Read the model definition and answer for the solid it produces. Units are mm, in the model's axes. Give positions to 0.01 mm unless a question says otherwise; leave off trailing zeros. Loops run counter-clockwise (first coordinate to the right, second up) from the corner with the lowest first, then second, coordinate; pieces in that order, holes last. Notation, with made-up numbers: (37, -6.75) -> (47, -6.75) arc R23 ccw to (47, 7.25) -> close; hole circle Ø4 at (5, 47). An arc over 180 degrees is marked (long way). One line per item, written item: value. Start each with the question number.
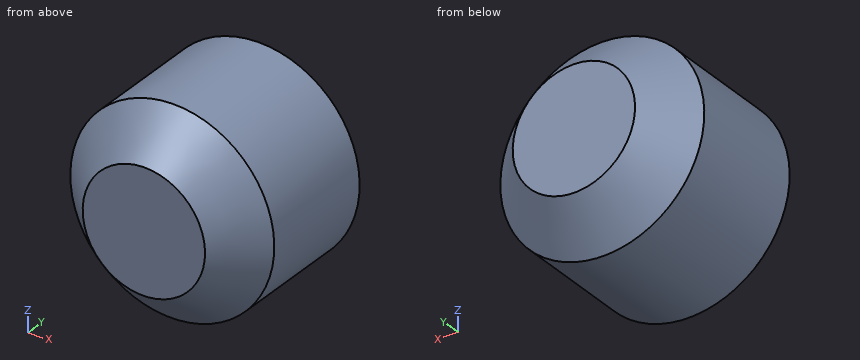
from build123d import *

# Parameters (mm, degrees)
SKETCH1_R           = 25
BOSS_EXTRUDE4_DEPTH = 50
CHAMFER2_SIZE       = 10
CHAMFER3_SIZE       = 10


with BuildPart() as part:
    # Sketch1 → Boss-Extrude4 (new body)
    with BuildSketch(Plane(origin=(0, 0, 0), x_dir=(1, 0, 0), z_dir=(0, 1, 0))):
        with Locations(Location((18.986456029, -23.441436424, 0), (0, 0, 270))):
            Circle(SKETCH1_R)
    extrude(amount=BOSS_EXTRUDE4_DEPTH)

    # Chamfer2
    chamfer2_edges = [part.edges().sort_by_distance(p)[0] for p in [
        (18.986456029, 50, -1.558563576),
    ]]
    chamfer(chamfer2_edges, length=CHAMFER2_SIZE)

    # Chamfer3
    chamfer3_edges = [part.edges().sort_by_distance(p)[0] for p in [
        (18.986456029, 0, -1.558563576),
    ]]
    chamfer(chamfer3_edges, length=CHAMFER3_SIZE)


solid = part.part
Item 1: Flat-ended cylindrical pins translate along their axes: pin 1 (4 mm diameter, centred on y = 38.5, z = 7.5, fed in from -X); pin 2 (5 mm diameter, centred on x = 6, y = 8, fed in from -Z); pin 3 (10 mm diameter, centred on x = 15.5, y = 30, fed in from +Z); pin 4 (2 mm diameter, centred on y = 14.5, z = 33, fed in from +X). Find the tip coordinate at first contact, or state that the pin passes through.
Item 2: Section A-A, the plane y = 44.5 is taken. Determine the outline of the cut face in (x, z).
Item 3: Consider L1, parallel to Z at x = 31.5, y = 8; L2, parallel to X at y = 6.5, z = 4; L3, parallel to X at y = 16.5, z = 3. Determine where each line is inside the solid, lowest interval first. Write a range as [from, to].
Item 4: Section B-B, the plane y = 22.5 is taken. Determine the outline of the cut face in (x, z).
Computed values:
1. pin 1: x = -1.77
1. pin 2: z = 1.24
1. pin 3: z = 48.44
1. pin 4: x = 42.48
2. outline: circle Ø41 at (18.99, 23.44)
3. L1: [4.14, 42.74]
3. L2: [9.81, 28.17]
3. L3: [4.59, 33.38]
4. outline: circle Ø50 at (18.99, 23.44)
